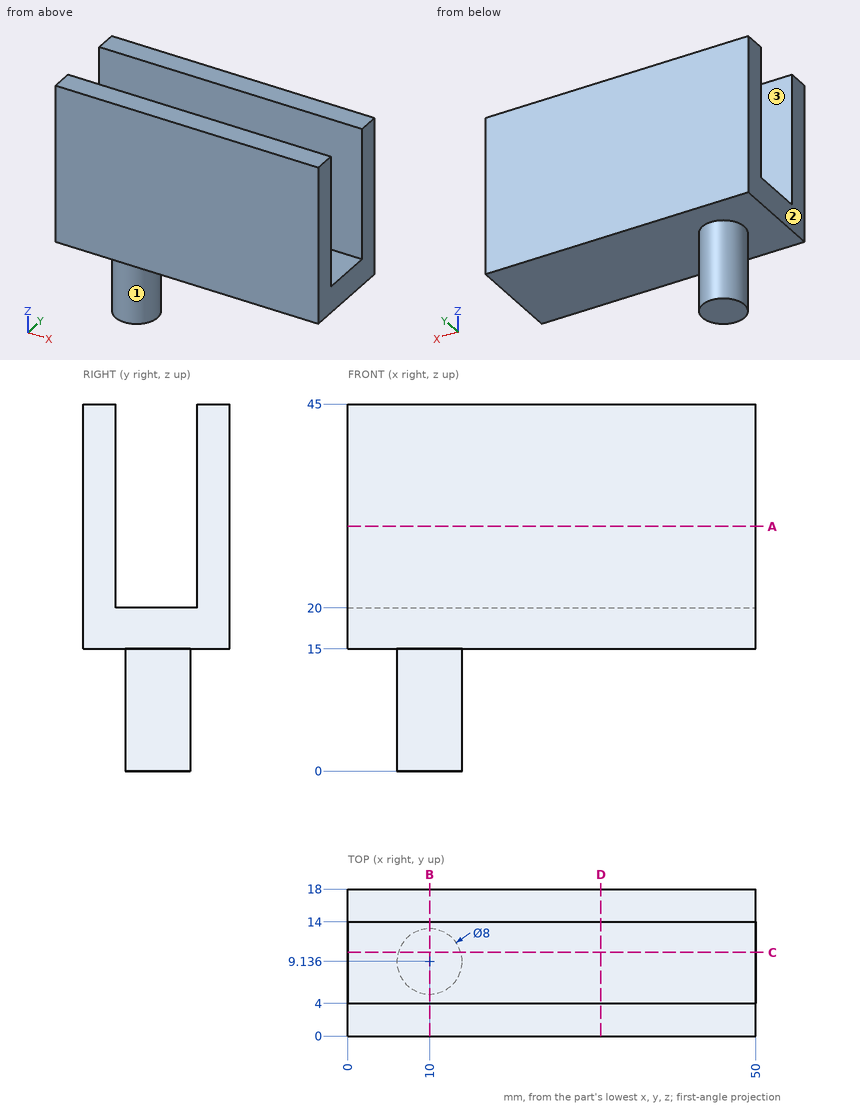
Print and shaded views of the part. All mm, measured from the part's lowest x, y and z. A direction names the side the tool comes from. Coordinates: 2 decimals unless noted, no trailing zeros. Order: outer loops, then holes, each group sorted by start corner. A loop starts at its lowest first (then second) coordinate and runs counter-clockwise, first axis right, second up. Notation, with made-up numbers: M 88,56.25 L 147,56.25 A34 ccw 147,88.25 Z; hole C -22.75,-31 d9. An arc over 180 degrees is marked long. Write each question's results on one line, items separated by ' | '. Start each with the question number.
Q1. Drill centre lines: probe 1 along Y at (x, z) = (19, 28); probe 2 along Z at (x, y) = (5, 16); probe 3 along Z at (x, y) = (27, 9.75). Where is each one in solid material? Low to high. Write a range as from..to.
Q2. Flat gauge pins, fed straight in: P1, Ø3, axis at y = 4.5, z = 12, coming from the +X side; P2, Ø6, axis at x = 34, y = 8, coming from the -Z side. Where does each tip first touch, or does it go through?
Q3. Cut at B-B (x = 10). List the corners of the cut face in (y, z).
Q4. Cut at A-A (z = 30). List the corners of the cut face in (x, y), then the cut area to 3 significant figures.
Q5. Cut at C-C (y = 10.25). List the corners of the cut face in (x, z), then the cut area to 3 significant figures.
Q6. Which spindle directions (+Z, -Z, +X, -X, +Y, -Y) get a long thin tool onto all of the face, cutting with end or side? Do the marked faces 1, 2 and 3. Say none if no direction does.
Q7. Cut at D-D (x = 31). List the corners of the cut face in (y, z), then the cut area to 3 significant figures.
Found:
1) probe 1: 0..4, 14..18 | probe 2: 15..45 | probe 3: 15..20
2) P1: x = 12.48 | P2: z = 15
3) outline: M 0,15 L 5.14,15 L 5.14,0 L 13.14,0 L 13.14,15 L 18,15 L 18,45 L 14,45 L 14,20 L 4,20 L 4,45 L 0,45 Z
4) outline: M 0,0 L 50,0 L 50,4 L 0,4 Z; M 0,14 L 50,14 L 50,18 L 0,18 Z | area: 400 mm²
5) outline: M 0,15 L 6.16,15 L 6.16,0 L 13.84,0 L 13.84,15 L 50,15 L 50,20 L 0,20 Z | area: 365 mm²
6) face 1: -Z | face 2: +Z, -Z, -X, +Y, -Y | face 3: +Z, +X, -X
7) outline: M 0,15 L 18,15 L 18,45 L 14,45 L 14,20 L 4,20 L 4,45 L 0,45 Z | area: 290 mm²
